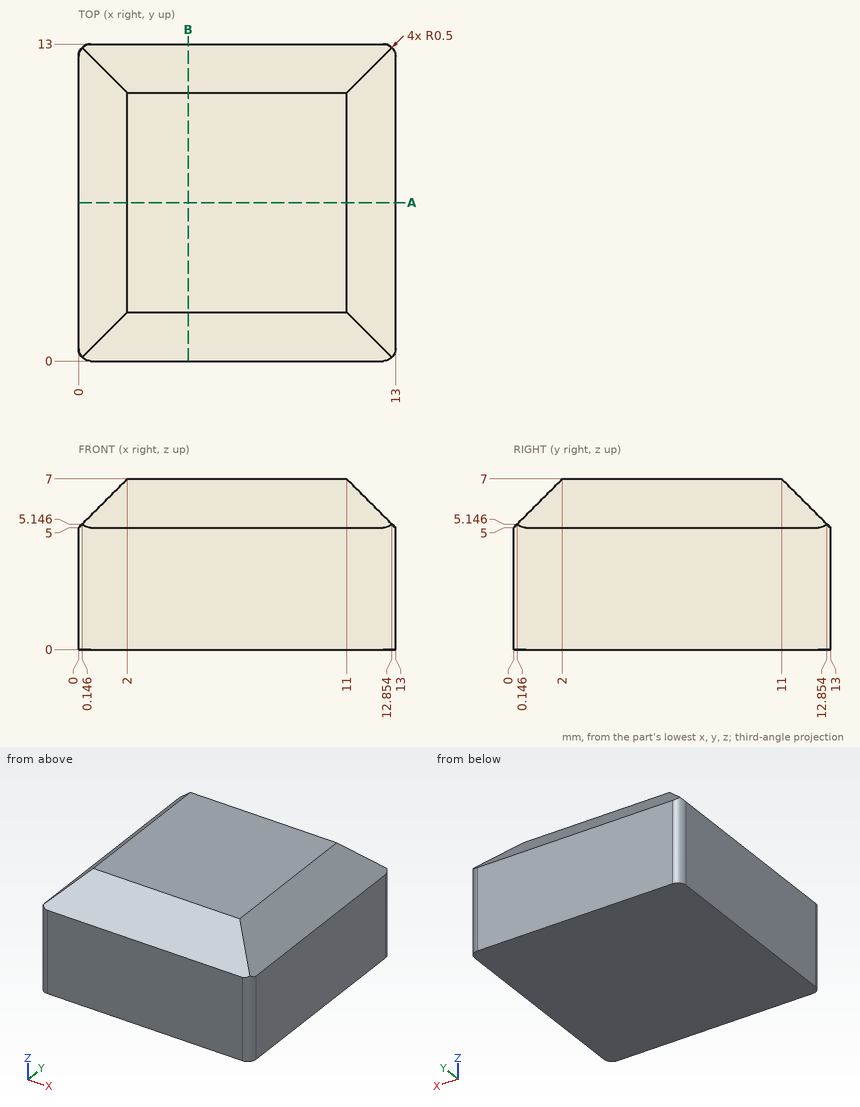
Verification items for this drawing (mm, ordinates from the low corner). Give positions to 0.01 mm unless a question says otherwise; leave off trailing zeros. Loops run counter-clockwise (first coordinate to the right, second up) from the corner with the lowest first, then second, coordinate; pieces in that order, holes last. Notation, with made-up numbers: M -33.75,-10 L 16.25,-10 A31 cw 16.25,25 Z; hole C 80.5,45.25 d9. An arc over 180 degrees is marked long. Answer as a JSON object with one key per item and string values. Group by question number.
Q1. Material ranges on line 1 along X through (y, z) = (6.25, 5.5); line 2 along Z through (x, y) = (4.25, 1.75); line 3 along Z through (x, y) = (7, 12.5), recorded low to high. Write a range as [from, to].
Q2. Cross-section at A-A on y = 6.5. Record the cut outline in (x, z).
Evaluation:
{
 "1": {"line 1": "x = [0.5, 12.5]", "line 2": "z = [0, 6.75]", "line 3": "z = [0, 5.5]"},
 "2": {"outline": "M 0,0 L 13,0 L 13,5 L 11,7 L 2,7 L 0,5 Z"}
}
